Source: CAD feature listing. Evaluate the final solid. Frame: model axes, mm. A direction names the side the tool comes from. Give positions to 0.01 mm unless a question says otherwise; leave off trailing zeros. Write each loop counter-clockwise with the first axis right and the second up, starting at its lowest first coordinate (ties: lowest second). Pieces come first, ordered by that corner, then holes. Notation, with made-up numbers: (69.25, -5.5) -> (82.25, -5.5) arc R25 ccw to (82.25, 30.5) -> close; hole circle Ø1 at (86, -24). An arc over 180 degrees is marked (long way). Write item = value, one per line.
from build123d import *

# Parameters (mm, degrees)
SKETCH1_W           = 133.35
SKETCH1_H           = 133.35
BOSS_EXTRUDE2_DEPTH = 3.175
SKETCH2_W           = 133.579746761
SKETCH2_H           = 133.57974676
SKETCH2_W_2         = 127
SKETCH2_H_2         = 127
EXTRUDE_THIN1_DEPTH = 76.2
BOSS_EXTRUDE3_START = -25.4
BOSS_EXTRUDE3_DEPTH = 3.175


with BuildPart() as part:
    # Sketch1 → Boss-Extrude2 (new body)
    with BuildSketch(Plane(origin=(0, 0, 0), x_dir=(1, 0, 0), z_dir=(0, 1, 0))):
        with Locations((-10.590734266, 10.501923077)):
            Rectangle(SKETCH1_W, SKETCH1_H)
    extrude(amount=BOSS_EXTRUDE2_DEPTH)

    # Sketch2 → Extrude-Thin1 (add)
    with BuildSketch(Plane(origin=(0, 3.175, 0), x_dir=(1, 0, 0), z_dir=(0, 1, 0))):
        with Locations((-10.590734266, 10.501923077)):
            Rectangle(SKETCH2_W, SKETCH2_H)
        with Locations((-10.590734266, 10.501923077)):
            Rectangle(SKETCH2_W_2, SKETCH2_H_2, mode=Mode.SUBTRACT)
    extrude(amount=EXTRUDE_THIN1_DEPTH)

    # Sketch4 → Boss-Extrude3 (add)
    with BuildSketch(Plane(origin=(0, 79.375, 0), x_dir=(1, 0, 0), z_dir=(0, 1, 0)).offset(BOSS_EXTRUDE3_START)):
        Polygon((-48.690734266, 74.001923077), (-74.090734266, 48.601923077), (-74.090734266, 74.001923077), align=None)
        Polygon((-74.090734266, -52.998076923), (-74.090734266, -27.598076923), (-48.690734266, -52.998076923), align=None)
        Polygon((52.909265734, 74.001923077), (27.509265734, 74.001923077), (52.909265734, 48.601923077), align=None)
        Polygon((52.909265734, -52.998076923), (52.909265734, -27.598076923), (27.509265734, -52.998076923), align=None)
    extrude(amount=-BOSS_EXTRUDE3_DEPTH)


solid = part.part
1) Material intervals for L1, parallel to X at y = 61, z = 27; L2, parallel to Z at x = 4, y = 36; L3, parallel to Y at x = -67, z = -68 (3 decimals), sorted ascending.
Computed:
L1 = -77.38 to -74.09, 52.91 to 56.2
L2 = -77.29 to -74, 53 to 56.29
L3 = 0 to 3.175, 50.8 to 53.975
2) Draft query along Y for faces 3 (the flat face through (46, 53.975, -67)), 4 (the flat face through (-67, 50.8, -67)), 5 (the flat face through (-12, 41, 56.288)). Return one class per face: pulls with the +Y half, pulls with the -Y half, needs draft (parallel to the pull), parting line crosses it, or undercut.
Computed:
face_3 = pulls with the +Y half
face_4 = undercut
face_5 = needs draft
3) Cut plane A-A (z = -27.5). Return the cut outline in (x, y) (3 decimals), then the cut area to 3 significant figures.
Computed:
outline = (-77.381, 3.175) -> (-77.266, 3.175) -> (-77.266, 0) -> (56.084, 0) -> (56.084, 3.175) -> (56.199, 3.175) -> (56.199, 79.375) -> (52.909, 79.375) -> (52.909, 3.175) -> (-74.091, 3.175) -> (-74.091, 79.375) -> (-77.381, 79.375) -> close
area = 925 mm²
4) Cut plane C-C (x = -39). Return the cut outline in (y, z) (3 decimals).
Computed:
outline = (0, -77.177) -> (3.175, -77.177) -> (3.175, -77.292) -> (79.375, -77.292) -> (79.375, -74.002) -> (3.175, -74.002) -> (3.175, 52.998) -> (79.375, 52.998) -> (79.375, 56.288) -> (3.175, 56.288) -> (3.175, 56.173) -> (0, 56.173) -> close
5) Access query for faces 1 (the flat face through (40.39, 52.41, 40.12)), 2 (the flat face through (46, 50.8, 46)). Directions: +Z, -Z, +X, -X, +Y, -Y. A direction counts if a zero-diameter tool reaches every point of the face in a straight line with its end or side. Return the directions, or none.
Computed:
face_1 = +Y
face_2 = none
6) Cut plane D-D (z = -60.5). Return the cut outline in (x, y) (3 decimals).
Computed:
outline = (-77.381, 3.175) -> (-77.266, 3.175) -> (-77.266, 0) -> (56.084, 0) -> (56.084, 3.175) -> (56.199, 3.175) -> (56.199, 79.375) -> (52.909, 79.375) -> (52.909, 53.975) -> (41.011, 53.975) -> (41.011, 50.8) -> (52.909, 50.8) -> (52.909, 3.175) -> (-74.091, 3.175) -> (-74.091, 50.8) -> (-62.193, 50.8) -> (-62.193, 53.975) -> (-74.091, 53.975) -> (-74.091, 79.375) -> (-77.381, 79.375) -> close
7) Contact query for flat-ended pins moving along their axis: pin 1 (2.5 mm diameter, centred on y = 1.5, z = 2, fed in from -X); pin 2 (1 mm diameter, centred on y = 2, z = -36, fed in from +X); pin 3 (12.5 mm diameter, centred on x = -58, z = -61, fed in from +Y) (3 decimals). Output: stop coordinate, or through.
Computed:
pin_1 = -77.27
pin_2 = 56.08
pin_3 = 53.975
8) Cut plane B-B (y = 32). Return the cut outline in (x, z), then the cut area to 3 significant figures.
Computed:
outline = (-77.38, -77.29) -> (56.2, -77.29) -> (56.2, 56.29) -> (-77.38, 56.29) -> close; hole (-74.09, -74) -> (52.91, -74) -> (52.91, 53) -> (-74.09, 53) -> close
area = 1,710 mm²
